Geometry: final body of the model. Coordinates: model frame, mm. A direction names the side the tool comes from. Give positions to 0.01 mm unless a question says otherwise; leave off trailing zeros. Order: outer loops, then holes, each group sorted by start corner. A loop starts at its lowest first (then second) coordinate and runs counter-clockwise, first axis right, second up. Notation, with made-up numbers: (-27, -33.75) -> (0, -33.75) arc R26 cw to (0, -10.75) -> close; hole circle Ø6 at (76, 73.25). An arc over 180 degrees is marked (long way). Answer in a Markdown table with one row per item. Add a question column.
Q1. Cut plane A-A on z = 10.5. Return the cut outline in (x, y), and give its area (3 significant figures).
Q2. Set-up query: faces 4 (the face through (2, 7.518, 3)), 5 (the face through (32, 8, 17)), 6 (the face through (-3.227, 12, 14)). Return all of +Z, -Z, +X, -X, +Y, -Y with unobstructed straight access to the full face (end or side cutting, diameter ignored); none if empty.
Q3. Line query: line 1 along X through (y, z) = (12.75, 7.5); line 2 along X through (y, z) = (6.25, 18.25); line 3 along X through (y, z) = (5.25, 5.75). Output: solid intervals per line, ascending. Write a range as from..to.
Q4. Contact query for flat-ended pins moving along their axis: P1, Ø1.8, axis at y = 13, z = 14, coming from the -X side; P2, Ø10, axis at x = -10.5, z = 10, coming from the +Y side; P3, Ø1, axis at y = 9, z = 13, coming from the +X side. Output: stop coordinate, or through.
Q5. Cut plane C-C on z = 18.75. Return the cut outline in (x, y), and give its area (3 significant figures).
Q6. Cut plane B-B on x = -1. Return the cut outline in (y, z).
Q7. Pull-direction query (X, two-part tool) for faces 1 (the face through (-21, 9.518, 11)), 2 (the face through (-22.325, 8.616, 0.855)), 3 (the face through (25.918, 8.616, 0.902)); classes: +X half, -X half, draft (parallel to the pull), parting line (faces both ways), or undercut.
Q8. Cut plane D-D on y = 14. Return the cut outline in (x, z), and give its area (3 significant figures).
from build123d import *

# Parameters (mm, degrees)
SKETCH_W        = 50
SKETCH_H        = 14
PAD_DEPTH       = 20
SKETCH001_W     = 48
SKETCH001_H     = 2
POCKET_DEPTH    = 18
SKETCH002_W     = 44
SKETCH002_H     = 4
POCKET001_DEPTH = 16
SKETCH003_W     = 16
SKETCH003_H     = 6
POCKET002_DEPTH = 18
SKETCH004_W     = 10
SKETCH004_H     = 3
POCKET003_DEPTH = 3
SKETCH005_W     = 14
SKETCH005_H     = 3
PAD001_DEPTH    = 8
SKETCH006_W     = 14
SKETCH006_H     = 3
PAD002_DEPTH    = 8
SKETCH007_R     = 1.5
POCKET004_DEPTH = 3
POCKET005_DEPTH = 3
SKETCH008_R     = 1.5
POCKET006_DEPTH = 3
FILLET_R        = 5
FILLET001_R     = 3
FILLET002_R     = 5
FILLET003_R     = 5
FILLET004_R     = 5
FILLET005_R     = 5


with BuildPart() as part:
    # Sketch → Pad (new body)
    with BuildSketch(Plane.XY):
        with Locations((1.773205, 8.517665)):
            Rectangle(SKETCH_W, SKETCH_H)
    extrude(amount=PAD_DEPTH)

    # Sketch001 (on Face6 of Pad) → Pocket (cut)
    with BuildSketch(Plane.XY.offset(20)):
        with Locations((1.773205, 8.517665)):
            Rectangle(SKETCH001_W, SKETCH001_H)
    extrude(amount=-POCKET_DEPTH, mode=Mode.SUBTRACT)

    # Sketch002 (on Face5 of Pocket) → Pocket001 (cut)
    with BuildSketch(Plane.XY.offset(20)):
        with Locations((1.773205, 5.517665)):
            Rectangle(SKETCH002_W, SKETCH002_H)
    extrude(amount=-POCKET001_DEPTH, mode=Mode.SUBTRACT)

    # Sketch003 (on Face5 of Pocket001) → Pocket002 (cut)
    with BuildSketch(Plane.XY.offset(20)):
        with Locations((-11.226795, 12.517665)):
            Rectangle(SKETCH003_W, SKETCH003_H)
        with Locations((14.773205, 12.517665)):
            Rectangle(SKETCH003_W, SKETCH003_H)
    extrude(amount=-POCKET002_DEPTH, mode=Mode.SUBTRACT)

    # Sketch004 (on Face8 of Pocket002) → Pocket003 (cut)
    with BuildSketch(Plane.XY.offset(20)):
        with Locations((1.773205, 11.017665)):
            Rectangle(SKETCH004_W, SKETCH004_H)
    extrude(amount=-POCKET003_DEPTH, mode=Mode.SUBTRACT)

    # Sketch005 (on Face12 of Pocket003) → Pad001 (join)
    with BuildSketch(Plane(origin=(-23.226795, 0, 0), x_dir=(0, -1, 0), z_dir=(-1, 0, 0))):
        with Locations((-8.517665, 18.5)):
            Rectangle(SKETCH005_W, SKETCH005_H)
    extrude(amount=PAD001_DEPTH)

    # Sketch006 (on Face3 of Pad001) → Pad002 (join)
    with BuildSketch(Plane.YZ.offset(26.773205)):
        with Locations((8.517665, 18.5)):
            Rectangle(SKETCH006_W, SKETCH006_H)
    extrude(amount=PAD002_DEPTH)

    # Sketch007 (on Face32 of Pad002) → Pocket004 (cut)
    with BuildSketch(Plane(origin=(0, 0, 17), x_dir=(1, 0, 0), z_dir=(0, 0, -1))):
        with Locations((-26.226795, -8.517665)):
            Circle(SKETCH007_R)
    extrude(amount=-POCKET004_DEPTH, mode=Mode.SUBTRACT)

    # Sketch007 (on Face32 of Pad002) → Pocket005 (cut)
    with BuildSketch(Plane(origin=(0, 0, 17), x_dir=(1, 0, 0), z_dir=(0, 0, -1))):
        with Locations((-26.226795, -8.517665)):
            Circle(SKETCH007_R)
    extrude(amount=-POCKET005_DEPTH, mode=Mode.SUBTRACT)

    # Sketch008 (on Face17 of Pocket005) → Pocket006 (cut)
    with BuildSketch(Plane.XY.offset(20)):
        with Locations((29.773205, 8.517665)):
            Circle(SKETCH008_R)
    extrude(amount=-POCKET006_DEPTH, mode=Mode.SUBTRACT)

    # Fillet
    fillet_edges = [part.edges().sort_by_distance(p)[0] for p in [
        (34.773205, 15.517665, 18.5),
        (34.773205, 1.517665, 18.5),
        (-31.226795, 1.517665, 18.5),
        (-31.226795, 15.517665, 18.5),
    ]]
    fillet(fillet_edges, radius=FILLET_R)

    # Fillet001
    fillet001_edges = [part.edges().sort_by_distance(p)[0] for p in [
        (-23.226795, 8.517665, 0),
        (26.773205, 8.517665, 0),
    ]]
    fillet(fillet001_edges, radius=FILLET001_R)

    # Fillet002
    fillet002_edges = [part.edges().sort_by_distance(p)[0] for p in [
        (-19.226795, 12.517665, 2),
    ]]
    fillet(fillet002_edges, radius=FILLET002_R)

    # Fillet003
    fillet003_edges = [part.edges().sort_by_distance(p)[0] for p in [
        (-3.226795, 12.517665, 2),
    ]]
    fillet(fillet003_edges, radius=FILLET003_R)

    # Fillet004
    fillet004_edges = [part.edges().sort_by_distance(p)[0] for p in [
        (22.773205, 12.517665, 2),
    ]]
    fillet(fillet004_edges, radius=FILLET004_R)

    # Fillet005
    fillet005_edges = [part.edges().sort_by_distance(p)[0] for p in [
        (6.773205, 12.517665, 2),
    ]]
    fillet(fillet005_edges, radius=FILLET005_R)


solid = part.part
Completed:
| question | item | result |
|---|---|---|
| 1 | outline | (-23.23, 1.52) -> (26.77, 1.52) -> (26.77, 15.52) -> (22.77, 15.52) -> (22.77, 9.52) -> (25.77, 9.52) -> (25.77, 7.52) -> (23.77, 7.52) -> (23.77, 3.52) -> (-20.23, 3.52) -> (-20.23, 7.52) -> (-22.23, 7.52) -> (-22.23, 9.52) -> (-19.23, 9.52) -> (-19.23, 15.52) -> (-23.23, 15.52) -> close; (-3.23, 9.52) -> (6.77, 9.52) -> (6.77, 15.52) -> (-3.23, 15.52) -> close |
| 1 | area | 236 mm² |
| 2 | face 4 | +Z |
| 2 | face 5 | -Z, +X, +Y, -Y |
| 2 | face 6 | +Z, +Y |
| 3 | line 1 | x = -23.23..-19.23, -3.23..6.77, 22.77..26.77 |
| 3 | line 2 | x = -31.22..-20.23, 23.77..34.77 |
| 3 | line 3 | x = -23.23..-20.23, 23.77..26.77 |
| 4 | P1 | stops at x = -23.23 |
| 4 | P2 | stops at y = 3.52 |
| 4 | P3 | stops at x = 26.77 |
| 5 | outline | (-31.23, 6.52) arc R5 ccw to (-26.23, 1.52) -> (29.77, 1.52) arc R5 ccw to (34.77, 6.52) -> (34.77, 10.52) arc R5 ccw to (29.77, 15.52) -> (22.77, 15.52) -> (22.77, 9.52) -> (25.77, 9.52) -> (25.77, 7.52) -> (23.77, 7.52) -> (23.77, 3.52) -> (-20.23, 3.52) -> (-20.23, 7.52) -> (-22.23, 7.52) -> (-22.23, 9.52) -> (-19.23, 9.52) -> (-19.23, 15.52) -> (-26.23, 15.52) arc R5 ccw to (-31.23, 10.52) -> close; (-3.23, 12.52) -> (6.77, 12.52) -> (6.77, 15.52) -> (-3.23, 15.52) -> close; hole circle Ø3 at (-26.23, 8.52); hole circle Ø3 at (29.77, 8.52) |
| 5 | area | 394 mm² |
| 6 | outline | (1.52, 0) -> (15.52, 0) -> (15.52, 20) -> (12.52, 20) -> (12.52, 17) -> (9.52, 17) -> (9.52, 2) -> (7.52, 2) -> (7.52, 4) -> (3.52, 4) -> (3.52, 20) -> (1.52, 20) -> close |
| 7 | face 1 | undercut |
| 7 | face 2 | -X half |
| 7 | face 3 | +X half |
| 8 | outline | (-29.81, 17) -> (-23.23, 17) -> (-23.23, 3) arc R3 ccw to (-20.23, 0) -> (23.77, 0) arc R3 ccw to (26.77, 3) -> (26.77, 17) -> (33.36, 17) -> (33.36, 20) -> (22.77, 20) -> (22.77, 7) arc R5 cw to (17.77, 2) -> (11.77, 2) arc R5 cw to (6.77, 7) -> (6.77, 20) -> (-3.23, 20) -> (-3.23, 7) arc R5 cw to (-8.23, 2) -> (-14.23, 2) arc R5 cw to (-19.23, 7) -> (-19.23, 20) -> (-29.81, 20) -> close |
| 8 | area | 481 mm² |
